Autodesk Inventor part; units mm, degrees
ref_plane "YZ Plane" through (0, 0, 0) normal (1, 0, 0) x (0, 1, 0)
ref_plane "XZ Plane" through (0, 0, 0) normal (0, 1, 0) x (-1, 0, 0)
ref_plane "XY Plane" through (0, 0, 0) normal (0, 0, 1) x (1, 0, 0)
sketch "Sketch1" plane through (0, 0, 0) normal (0, 0, 1) x (1, 0, 0)
  line L0 (0, 0) -> (15, 0)
  line L1 (15, 0) -> (15, 15)
  line L2 (15, 15) -> (0, 15)
  line L3 (0, 15) -> (0, 0)
  dimension "d0" = 15
  dimension "d1" = 15
extrude "Extrusion1" add sketch "Sketch1" along normal blind 40
sketch "Sketch2" plane through (0, 0, 0) normal (0, 0, -1) x (-1, 0, 0)
  circle A0 centre (-7.5, 7.5) radius 7.5
  line L0 (-15, 15) -> (0, 15)
  line L1 (0, 15) -> (0, 0)
  line L2 (0, 0) -> (-15, 0)
  line L3 (-15, 0) -> (-15, 15)
  line L4 (-15, 15) -> (0, 15)
  line L5 (0, 0) -> (-15, 0)
  line L6 (0, 15) -> (0, 0)
  line L7 (-15, 0) -> (-15, 15)
extrude "Extrusion2" cut sketch "Sketch2" against normal blind 5 contours L1 L2 A0 | A0 L0 L1 | A0 L3 L0 | L2 L3 A0
properties part number "EF-Arm"
Check sheet for the modelled part. Datum: model origin and axes. Units: mm. A direction names the side the tool comes from. Give positions to 0.01 mm unless a question says otherwise; leave off trailing zeros. Loops run counter-clockwise (first coordinate to the right, second up) from the corner with the lowest first, then second, coordinate; pieces in that order, holes last. Notation, with made-up numbers: M 26,63 L 64,63 A29 ccw 64,87 Z; hole C 1,66.25 d4. An arc over 180 degrees is marked long. Answer in a Markdown table with one row per item.
1) Cross-section at C-C (y = 12.5). Enter the section's corners in (x, z).
Solutions:
| item | result |
|---|---|
| outline | M 0,5 L 1.91,5 L 1.91,0 L 13.09,0 L 13.09,5 L 15,5 L 15,40 L 0,40 Z |
2) Thickness scan on line 1 (Z direction, x = 1, y = 14.25); line 2 (Y direction, x = 1.5, z = 4); line 3 (X direction, y = 8.5, z = 3). Record the ranges inside material, lowest first.
Solutions:
| item | result |
|---|---|
| line 1 | z = 5 to 40 |
| line 2 | y = 3 to 12 |
| line 3 | x = 0.07 to 14.93 |
3) Cross-section at B-B (z = 3). Enter the section's corners in (x, y).
Solutions:
| item | result |
|---|---|
| outline | C 7.5,7.5 d15 |
4) Tool access check on faces 1 (the face through (2, 2, 5)), 2 (the face through (2, 13, 5)), 3 (the face through (9.13, 0.18, 2.46)), 4 (the face through (13, 2, 5)), 5 (the face through (13, 13, 5)). Record the directions out of +Z, -Z, +X, -X, +Y, -Y that give a thin tool (end or side, any length) a straight path to the whole face; none if there is none.
Solutions:
| item | result |
|---|---|
| face 1 | -Z, -X, -Y |
| face 2 | -Z, -X, +Y |
| face 3 | -Z |
| face 4 | -Z, +X, -Y |
| face 5 | -Z, +X, +Y |
5) Cross-section at A-A (y = 3). Enter the section's corners in (x, z).
Solutions:
| item | result |
|---|---|
| outline | M 0,5 L 1.5,5 L 1.5,0 L 13.5,0 L 13.5,5 L 15,5 L 15,40 L 0,40 Z |
